Here's the drawing with two shaded views (mm, measured from the low corner). I have some questions. A direction names the side the tool comes from. Round coordinates to 2 decimals unless told otherwise and drop trailing zeros. Write each loop counter-clockwise with the first axis right and the second up, starting at its lowest first coordinate (ties: lowest second). Pieces come first, ordered by that corner, then holes. Notation, with made-up numbers: (8.25, 3.25) - (61.25, 3.25) arc R6 cw to (61.25, 14.25) - close; hole circle Ø9 at (46, -5). An arc over 180 degrees is marked (long way). Return JSON: item names as keys, results as strings. Group by question number.
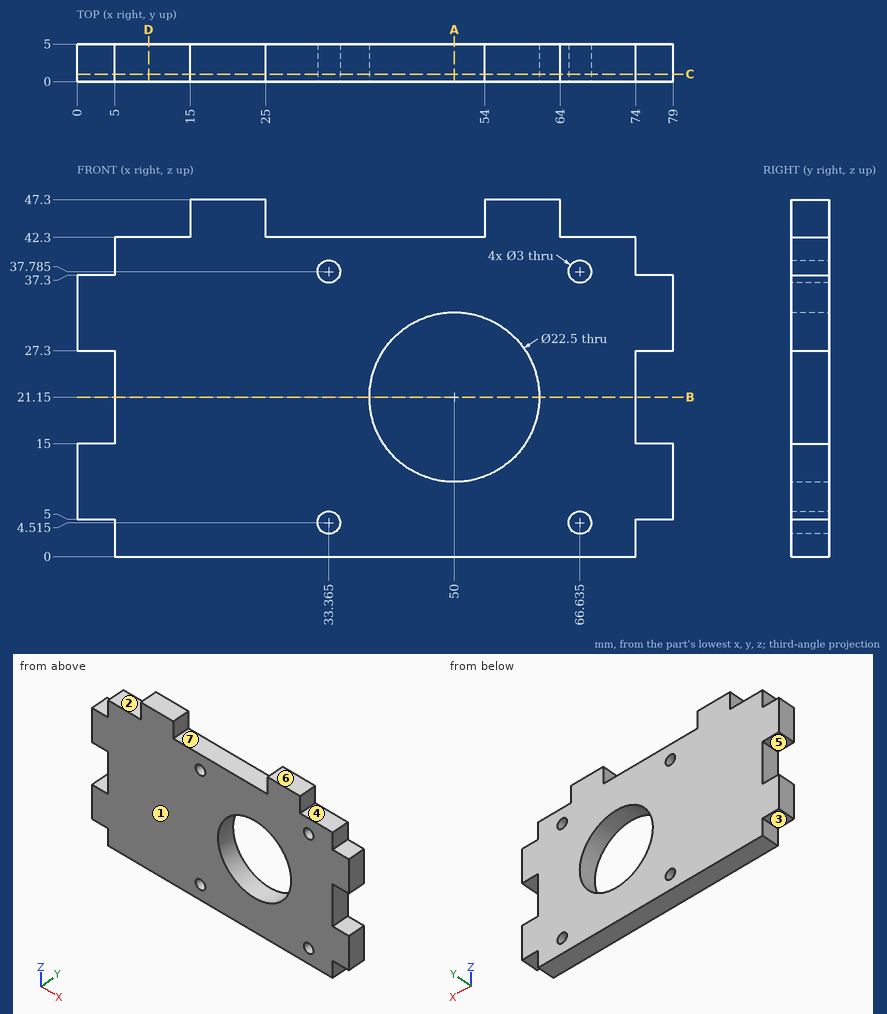
1) Imagine slicing it at A-A (x = 50). Please give me the cut outline in (y, z).
2) I need wall thicknesses on line 1 along X through (y, z) = (3.4, 44.5); line 2 along Z through (x, y) = (4, 4.2); line 3 along Z through (x, y) = (70.5, 2.65). Which ranges of each line are inside material? Lowest first, please.
3) Imagine slicing it at D-D (x = 9.5). Please give me the cut outline in (y, z).
4) Imagine slicing it at B-B (z = 21.15). Please give me the cut outline in (x, y).
5) Imagine slicing it at C-C (y = 1). Give the number of separate pieces and of enclosed holes in the cut face, plus the area to 3 significant figures.
6) If we mould it in two halves opening along X, with no side actions, what happens to the marked faces 6 and 7? For each: released by +X, released by -X, zero draft, split by the parting line, or undercut.
7) For the marked faces 1, 2, 3, 4 and 5, which set-ups out of +Z, -Z, +X, -X, +Y, -Y let a thin tool reach every point of the face, with its end or its side?
8) Will these pins go through, and if not, where does the flat tip stop? pin 1 Ø2.5 at (x, y) = (76.5, 2) entering from +Z; pin 2 Ø2.5 at (y, z) = (1.5, 40.5) entering from -X; pin 3 Ø2.5 at (y, z) = (2.5, 45) entering from -X.
Results found:
{
 "1": {"outline": "(0, 0) - (5, 0) - (5, 9.9) - (0, 9.9) - close; (0, 32.4) - (5, 32.4) - (5, 42.3) - (0, 42.3) - close"},
 "2": {"line 1": "x = 15 to 25, 54 to 64", "line 2": "z = 5 to 15, 27.3 to 37.3", "line 3": "z = 0 to 42.3"},
 "3": {"outline": "(0, 0) - (5, 0) - (5, 42.3) - (0, 42.3) - close"},
 "4": {"outline": "(5, 0) - (38.75, 0) - (38.75, 5) - (5, 5) - close; (61.25, 0) - (74, 0) - (74, 5) - (61.25, 5) - close"},
 "5": {"separate pieces": "1", "enclosed holes": "5", "area": "2,790 mm²"},
 "6": {"face 6": "zero draft", "face 7": "undercut"},
 "7": {"face 1": "+Z, -Z, +X, -X, -Y", "face 2": "+Z, -X, +Y, -Y", "face 3": "-Z, -X, +Y, -Y", "face 4": "+Z, +X, +Y, -Y", "face 5": "-X, +Y, -Y"},
 "8": {"pin 1": "stops at z = 37.3", "pin 2": "stops at x = 5", "pin 3": "stops at x = 15"}
}
